```python
from build123d import *

# Parameters (mm, degrees)
BOSS_EXTRUDE1_DEPTH = 6
SKETCH4_R           = 3.57
BOSS_EXTRUDE2_DEPTH = 1.27
SKETCH3_R           = 2.5
CUT_EXTRUDE1_DEPTH  = 10.439442655
SKETCH5_R           = 1
CUT_EXTRUDE3_DEPTH  = 0.15


with BuildPart() as part:
    # Sketch2 → Boss-Extrude1 (new body)
    with BuildSketch(Plane(origin=(0, 0, 0), x_dir=(0, 0, -1), z_dir=(1, 0, 0))):
        Polygon((3.919437566, -2.29861752), (3.950379949, 2.245023741), (0.030942383, 4.54364126), (-3.919437566, 2.29861752), (-3.950379949, -2.245023741), (-0.030942383, -4.54364126), align=None)
    extrude(amount=BOSS_EXTRUDE1_DEPTH)

    # Sketch4 → Boss-Extrude2 (add)
    with BuildSketch(Plane.ZY):
        with Locations(Location((0, 0, 0), (0, 0, 180))):
            Circle(SKETCH4_R)
    extrude(amount=BOSS_EXTRUDE2_DEPTH)

    # Sketch3 → Cut-Extrude1 (cut, through all)
    with BuildSketch(Plane.ZY.offset(1.27)):
        with Locations((0.79, 0)):
            Circle(SKETCH3_R)
    extrude(amount=-CUT_EXTRUDE1_DEPTH, mode=Mode.SUBTRACT)

    # Sketch5 → Cut-Extrude3 (cut)
    with BuildSketch(Plane(origin=(0, 0.02679689, 3.934908757), x_dir=(1, 0, 0), z_dir=(0, -0.006809882993303443, -0.9999768124779782))):
        with Locations(Location((3, 0, 0), (0, 0, 90))):
            Circle(SKETCH5_R)
    extrude(amount=CUT_EXTRUDE3_DEPTH, mode=Mode.SUBTRACT)


solid = part.part
```
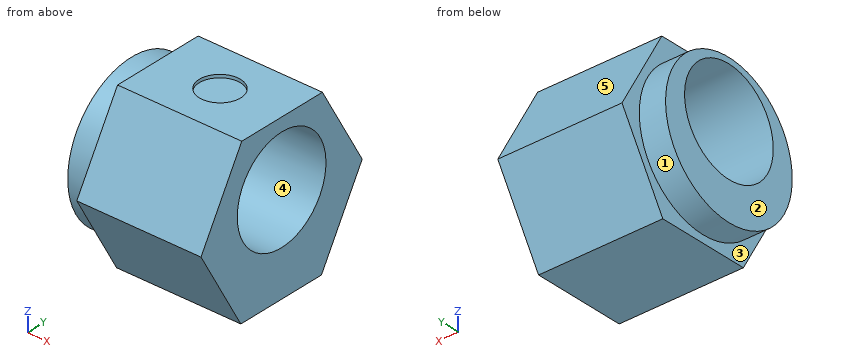
Could you check a few things on this model? Use its own coordinates, in mm. Face numbers are marked on the shaded views. A direction names the side the tool comes from. Give positions to 0.01 mm unless a question says otherwise; leave off trailing zeros. Loops run counter-clockwise (first coordinate to the right, second up) from the corner with the lowest first, then second, coordinate; pieces in that order, holes last. Notation, with made-up numbers: (19.25, 43.5) - (48.25, 43.5) arc R7 ccw to (48.25, 47.5) - close; hole circle Ø5 at (22.5, -24.5). An arc over 180 degrees is marked (long way). Answer in a Markdown table with one row per item. Add a question column.
Q1. We'd pull the mould along Z, two halves only. Please class the marked faces 3, 4 and 5: +Z half, -Z half, draft (parallel to the pull), parting line (faces both ways), or undercut.
Q2. Which directions (+Z, -Z, +X, -X, +Y, -Y) give clear straight access to the entire face, cutting with the end or side of a thin tool? Please do the marked faces 1 and 2.
Q3. If we section it at B-B (z = 0.79): List the corners of the cut face in (x, y) for me.
Q4. If we section it at D-D (y = 3): List the corners of the cut face in (x, z) for me.
Q5. For pin 1 (4 mm diameter, centred on x = 4.5, y = 2.5, fed in from +Z); pin 2 (1.5 mm diameter, centred on x = 4.5, y = 3.5, fed in from -Z), each with a flat end and sliding along its axis, tell me the tip position at first contact or that it passes through.
Q6. If we section it at C-C (z = -2.25): List the corners of the cut face in (x, y) for me.
Q7. If we section it at A-A (y = -2): List the corners of the cut face in (x, z) for me.
Q8. Please list where these lines run through material, in increasing order: L1, parallel to X at y = 3, z = -2; L2, parallel to Y at x = 5.75, z = 3; L3, parallel to Z at x = 1, y = 1.5. Write a range as from..to.
The answers:
| question | item | result |
|---|---|---|
| 1 | face 3 | draft |
| 1 | face 4 | undercut |
| 1 | face 5 | +Z half |
| 2 | face 1 | -X |
| 2 | face 2 | +Z, -Z, -X, +Y, -Y |
| 3 | outline | (-1.27, -3.48) - (0, -3.48) - (0, -4.1) - (6, -4.1) - (6, -2.5) - (-1.27, -2.5) - close; (-1.27, 2.5) - (6, 2.5) - (6, 4.08) - (0, 4.08) - (0, 3.48) - (-1.27, 3.48) - close |
| 4 | outline | (-1.27, -1.94) - (0, -1.94) - (0, -2.66) - (6, -2.66) - (6, 2.69) - (0, 2.69) - (0, 1.94) - (-1.27, 1.94) - close |
| 5 | pin 1 | stops at z = 3.93 |
| 5 | pin 2 | stops at z = -3.09 |
| 6 | outline | (-1.27, -2.77) - (0, -2.77) - (0, -3.25) - (6, -3.25) - (6, 3.24) - (0, 3.24) - (0, 2.77) - (-1.27, 2.77) - close |
| 7 | outline | (-1.27, -2.96) - (0, -2.96) - (0, -3.92) - (6, -3.92) - (6, -0.71) - (-1.27, -0.71) - close; (-1.27, 2.29) - (6, 2.29) - (6, 3.95) - (0, 3.95) - (0, 2.96) - (-1.27, 2.96) - close |
| 8 | L1 | x = 0..6 |
| 8 | L2 | y = -2.8..-1.17, 1.17..2.82 |
| 8 | L3 | z = -3.95..-1.21, 2.79..3.92 |
